Geometry check sheet. Reference: the model listing, model coordinates, mm. Round coordinates to 2 decimals unless told otherwise and drop trailing zeros. Order: outer loops, then holes, each group sorted by start corner. A loop starts at its lowest first (then second) coordinate and runs counter-clockwise, first axis right, second up. Notation, with made-up numbers: (-36.5, -10.5) - (-5.5, -10.5) arc R25 ccw to (-5.5, 20.5) - close; hole circle Ø5 at (18, 6.5). An arc over 180 degrees is marked (long way). Use a Markdown table: item, result. Add a question column.
(1) Section check A-A on z = 5.5. Record the boundary of the cut face in (x, y).
(2) Gauge pin test, flat ends, axial feed: P1, Ø2, axis at y = -4.5, z = 4, coming from the +X side; P2, Ø4, axis at y = 7, z = 1.5, coming from the -X side; P3, Ø1.5, axis at x = 6.5, z = 6, coming from the +Y side. Record the tip position at first contact, or that the pin passes through.
(3) Mould release check, pull along X, two halves, no side actions. Record for faces 1 (the face through (-2.17, -9.76, 3.95)), 2 (the face through (7.39, -3.06, 3.96)): released by +X, released by -X, zero draft, split by the parting line, or undercut.
(4) Thickness scan on line 1 along Y through (x, z) = (0, 4.55); line 2 along X through (y, z) = (3.5, 5.75); line 3 along Y through (x, z) = (-6.75, 4.5). Record the ranges inside material, lowest first. Write a range as [from, to].
```python
from build123d import *

# Parameters (mm, degrees)
F2_R     = 10
F2_R_2   = 8
F3_DEPTH = 8
F4_R     = 0.6666666667
F6_R     = 0.6666666667


# Not quite as in the source:
# - a fillet or chamfer that OpenCascade refuses, or shapes differently, is made with other operations: its cross-section is extruded or revolved along the edge and cut away or added


with BuildPart() as f3:
    # F2 (on Top) → F3 (new body)
    with BuildSketch(Plane.XY):
        Circle(F2_R)
        Circle(F2_R_2, mode=Mode.SUBTRACT)
    extrude(amount=F3_DEPTH)

    # F4
    f4_edges = [f3.edges().sort_by_distance(p)[0] for p in [
        (-10, 0, 8),
        (-10, 0, 0),
    ]]
    fillet(f4_edges, radius=F4_R)

    # F5: chamfer of 2 x 0.6666666667 on 2 edges, made by hand

    # F5_s1 → F5_t2 (revolve, cut)
    with BuildSketch(Plane.XZ):
        Polygon((10, 0), (8, 0.6666666667), (8, 0), align=None)
    revolve(axis=Axis((0, 0, 0), (0, 0, 1)), mode=Mode.SUBTRACT)

    # F5_s3 → F5_t4 (revolve, cut)
    with BuildSketch(Plane.XZ):
        Polygon((10, 8), (8, 7.3333333333), (8, 8), align=None)
    revolve(axis=Axis((0, 0, 8), (0, 0, 1)), mode=Mode.SUBTRACT)

    # F6
    f6_edges = [f3.edges().sort_by_distance(p)[0] for p in [
        (-8, 0, 7.333333),
        (-8, 0, 0.666667),
    ]]
    fillet(f6_edges, radius=F6_R)


solid = f3.part
```
Check sheet entries:
| question | item | result |
|---|---|---|
| 1 | outline | circle Ø20 at (0, 0); hole circle Ø16 at (0, 0) |
| 2 | P1 | stops at x = 9.37 |
| 2 | P2 | stops at x = -8.66 |
| 2 | P3 | stops at y = 8.18 |
| 3 | face 1 | split by the parting line |
| 3 | face 2 | undercut |
| 4 | line 1 | y = [-10, -8], [8, 10] |
| 4 | line 2 | x = [-9.37, -7.19], [7.19, 9.37] |
| 4 | line 3 | y = [-7.38, -4.29], [4.29, 7.38] |
